Autodesk Inventor part; units mm, degrees
ref_plane "YZ Plane" through (0, 0, 0) normal (1, 0, 0) x (0, 1, 0)
ref_plane "XZ Plane" through (0, 0, 0) normal (0, 1, 0) x (-1, 0, 0)
ref_plane "XY Plane" through (0, 0, 0) normal (0, 0, 1) x (1, 0, 0)
sketch "Esquisse1" plane through (0, 0, 0) normal (1, 0, 0) x (0, 1, 0)
  line L0 (0, 21.0755) -> (0, -24.2543)
  line L1 (7.85, -1.5) -> (7.85, 0)
  line L2 (7.85, 0) -> (11, 0)
  line L3 (11, 0) -> (11, -6)
  line L4 (11, -6) -> (7.85, -6)
  line L5 (7.85, -6) -> (7.85, -4.5)
  line L6 (7.85, -4.5) -> (5.85, -4.5)
  line L7 (5.85, -4.5) -> (5.85, -12)
  line L8 (5.85, -12) -> (4, -12)
  line L9 (7.85, -1.5) -> (5.85, -1.5)
  line L10 (5.85, -1.5) -> (5.85, 0)
  line L11 (5.85, 0) -> (4, 0)
  line L12 (4, 0) -> (4, -12)
  line L13 (6.85, -1.5) -> (6.85, -4.5) construction
  line L14 (6.85, -3) -> (11, -3) construction
  point P0 (0, 0)
  point P1 (7.85, -5.25)
  dimension "d0" = 11.7
  dimension "d1" = 8
  dimension "d2" = 12
  dimension "d3" = 6
  dimension "d4" = 22
  dimension "d5" = 2
  dimension "d6" = 3
revolve "Révolution1" add sketch "Esquisse1" angle 360 about axis through (0, 0, 21.0755) along (0, 0, -1)
properties part number "engrenage_simplifie_nouveau"
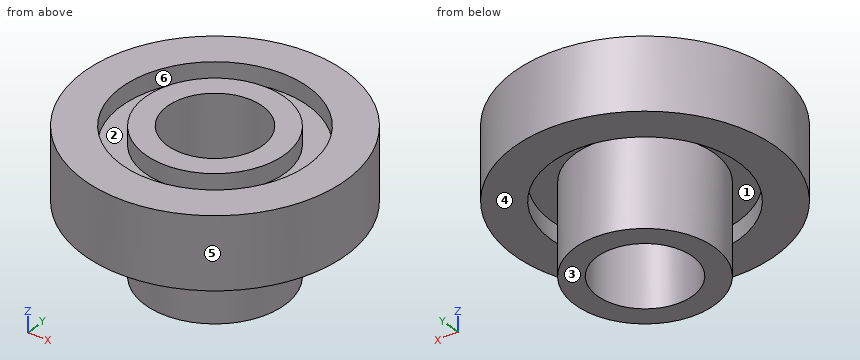
For this review, take the finished solid that the model builds, in its own axes (mm). Face numbers are marked on the shaded views. A direction names the side the tool comes from. Round coordinates to 2 decimals unless told otherwise and drop trailing zeros. Loops run counter-clockwise (first coordinate to the right, second up) from the corner with the lowest first, then second, coordinate; pieces in that order, holes last. Notation, with made-up numbers: (40.25, 66) - (76.25, 66) arc R8 ccw to (76.25, 78) - close; hole circle Ø6 at (75, 61). An arc over 180 degrees is marked (long way). One line per item, written item: value. Start each with the question number.
Item 1: Take a section at B-B (y = 3.5). Give the boundary of the cut face in (x, z).
Item 2: The part is to be moulded in two halves that separate along Y. For the marked faces 4, 5 and 6, say which applies: +Y half, -Y half, draft (parallel to the pull), parting line (faces both ways), or undercut.
Item 3: Take a section at D-D (x = 7). Give the boundary of the cut face in (y, z), plus the area to 3 significant figures.
Item 4: Take a section at C-C (z = -2.5). Give the boundary of the cut face in (x, y).
Item 5: For the marked faces 1, 2 and 3, list the 3-axis set-ups (+Z, -Z, +X, -X, +Y, -Y) from which the entire face can be reached by the end or side of a thin tool; tool diameter is ignored.
Item 6: Take a section at A-A (x = 0). Give the boundary of the cut face in (y, z).
Item 7: For L1, parallel to X at y = 0, z = -5.6; L2, parallel to X at y = 0, z = -7; L3, parallel to Z at x = 7.5, y = 3, list the stretches that pass through material, from the lowest coordinate up.
Item 8: Clearance check with flat-ended pins moving along their axes: pin 1 Ø3 at (x, z) = (-6, -9.5) entering from -Y; pin 2 Ø1.5 at (x, z) = (-3, -10.5) entering from -Y; pin 3 Ø6 at (x, z) = (6.5, -4.5) entering from +Y; pin 4 Ø6.5 at (x, y) = (0, 0) entering from -Z. State where each tip first meets the part, or that it passes through.
Answer below:
1. outline: (-10.43, -6) - (-7.03, -6) - (-7.03, -4.5) - (-4.69, -4.5) - (-4.69, -12) - (-1.94, -12) - (-1.94, 0) - (-4.69, 0) - (-4.69, -1.5) - (-7.03, -1.5) - (-7.03, 0) - (-10.43, 0) - close; (1.94, -12) - (4.69, -12) - (4.69, -4.5) - (7.03, -4.5) - (7.03, -6) - (10.43, -6) - (10.43, 0) - (7.03, 0) - (7.03, -1.5) - (4.69, -1.5) - (4.69, 0) - (1.94, 0) - close
2. face 4: draft
2. face 5: parting line
2. face 6: undercut
3. outline: (-8.49, -6) - (-3.55, -6) - (-3.55, -4.5) - (3.55, -4.5) - (3.55, -6) - (8.49, -6) - (8.49, 0) - (3.55, 0) - (3.55, -1.5) - (-3.55, -1.5) - (-3.55, 0) - (-8.49, 0) - close
3. area: 80.5 mm2
4. outline: circle Ø22 at (0, 0); hole circle Ø8 at (0, 0)
5. face 1: -Z
5. face 2: +Z
5. face 3: -Z, +X, -X, +Y, -Y
6. outline: (-11, -6) - (-7.85, -6) - (-7.85, -4.5) - (-5.85, -4.5) - (-5.85, -12) - (-4, -12) - (-4, 0) - (-5.85, 0) - (-5.85, -1.5) - (-7.85, -1.5) - (-7.85, 0) - (-11, 0) - close; (4, -12) - (5.85, -12) - (5.85, -4.5) - (7.85, -4.5) - (7.85, -6) - (11, -6) - (11, 0) - (7.85, 0) - (7.85, -1.5) - (5.85, -1.5) - (5.85, 0) - (4, 0) - close
7. L1: x = -11 to -7.85, -5.85 to -4, 4 to 5.85, 7.85 to 11
7. L2: x = -5.85 to -4, 4 to 5.85
7. L3: z = -6 to 0
8. pin 1: stops at y = -3.74
8. pin 2: stops at y = -5.4
8. pin 3: stops at y = 10.43
8. pin 4: passes through
